Could you check a few things on this drawing? It's one solid part, dimensions in mm from its lowest x, y, z. Coordinates: 2 decimals unless noted, no trailing zeros. Write each loop counter-clockwise with the first axis right and the second up, starting at its lowest first coordinate (ties: lowest second). Pieces come first, ordered by that corner, then holes. Notation, with made-up numbers: (0.5, 77) - (23.5, 77) arc R19 cw to (23.5, 104) - close; hole circle Ø11 at (78.5, -28.5). An arc over 180 degrees is marked (long way). Answer as a JSON object with one key per item and string values. Group by question number.
1) If we section it at A-A (x = 56): Write out the boundary of the cut face in (y, z).
2) If we section it at B-B (y = 30): Write out the boundary of the cut face in (x, z).
3) We'd pull the mould along Y, two halves only. Please class the marked faces 1, 2 and 3: released by +Y, released by -Y, zero draft, split by the parting line, or undercut.
4) Will these pins go through, and if not, where does the flat tip stop? pin 1 Ø8 at (x, y) = (28, 30.5) entering from +Z; pin 2 Ø5 at (x, y) = (44, 23.5) entering from +Z; pin 3 Ø12 at (x, z) = (16.5, 16.5) entering from -Y; pin 4 Ø1.6 at (x, y) = (56, 56) entering from +Z.
5) Please list where these lines run through material, in increasing order: line 1 along Y through (x, z) = (4, 1); line 2 along Y through (x, z) = (30, 1); line 3 along Z through (x, y) = (29, 7).
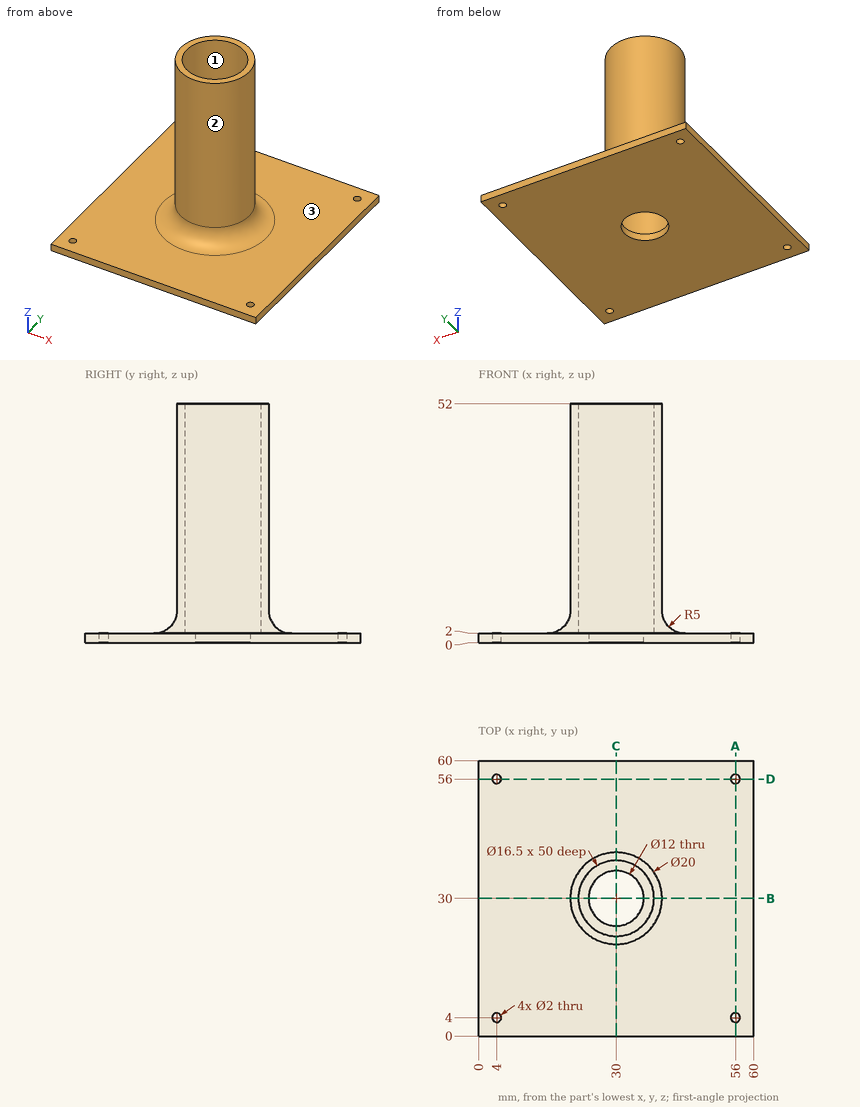
Here are the results:
{
 "1": {"outline": "(0, 0) - (3, 0) - (3, 2) - (0, 2) - close; (5, 0) - (55, 0) - (55, 2) - (5, 2) - close; (57, 0) - (60, 0) - (60, 2) - (57, 2) - close"},
 "2": {"outline": "(0, 0) - (24, 0) - (24, 2) - (21.75, 2) - (21.75, 52) - (20, 52) - (20, 7) arc R5 cw to (15, 2) - (0, 2) - close; (36, 0) - (60, 0) - (60, 2) - (45, 2) arc R5 cw to (40, 7) - (40, 52) - (38.25, 52) - (38.25, 2) - (36, 2) - close"},
 "3": {"face 1": "undercut", "face 2": "split by the parting line", "face 3": "zero draft"},
 "4": {"pin 1": "stops at z = 2", "pin 2": "stops at z = 2.45", "pin 3": "stops at y = 23.39", "pin 4": "passes through"},
 "5": {"line 1": "y = 0 to 3, 5 to 55, 57 to 60", "line 2": "y = 0 to 24, 36 to 60", "line 3": "z = 0 to 2"}
}
